```python
from build123d import *

# Parameters (mm, degrees)
F0_R     = 45.212
F1_DEPTH = 12.065
F2_R     = 2.5908
F3_DEPTH = 25.4
F4_R     = 14.5415
F5_DEPTH = 25.4
F6_R     = 6.731
F7_DEPTH = 9.525


with BuildPart() as f1:
    # F0 (on Top) → F1 (new body)
    with BuildSketch(Plane.XY):
        Circle(F0_R)
    extrude(amount=F1_DEPTH)

    # F2 (on face) → F3 (cut)
    with BuildSketch(Plane.XY.offset(12.065)):
        with Locations((-6.163129, 23.001109)):
            Circle(F2_R)
        with Locations((-23.001109, 6.163129)):
            Circle(F2_R)
        with Locations((-16.83798, -16.83798)):
            Circle(F2_R)
        with Locations((6.163129, -23.001109)):
            Circle(F2_R)
        with Locations((23.001109, -6.163129)):
            Circle(F2_R)
        with Locations((16.83798, 16.83798)):
            Circle(F2_R)
    extrude(amount=-F3_DEPTH, mode=Mode.SUBTRACT)

    # F4 (on face) → F5 (cut)
    with BuildSketch(Plane.XY.offset(12.065)):
        Circle(F4_R)
    extrude(amount=-F5_DEPTH, mode=Mode.SUBTRACT)

    # F6 (on face) → F7 (cut)
    with BuildSketch(Plane.XY.offset(12.065)):
        with Locations((-6.163129, 23.001109)):
            Circle(F6_R)
        with Locations((16.83798, 16.83798)):
            Circle(F6_R)
        with Locations((23.001109, -6.163129)):
            Circle(F6_R)
        with Locations((6.163129, -23.001109)):
            Circle(F6_R)
        with Locations((-16.83798, -16.83798)):
            Circle(F6_R)
        with Locations((-23.001109, 6.163129)):
            Circle(F6_R)
    extrude(amount=-F7_DEPTH, mode=Mode.SUBTRACT)


solid = f1.part
```
Could you check a few things on this model? Use its own coordinates, in mm. A direction names the side the tool comes from. Round coordinates to 2 decimals unless told otherwise and drop trailing zeros. Order: outer loops, then holes, each group sorted by start corner. A loop starts at its lowest first (then second) coordinate and runs counter-clockwise, first axis right, second up. Notation, with made-up numbers: (8.5, -2.75) -> (67.5, -2.75) arc R16 cw to (67.5, 3.25) -> close; hole circle Ø4 at (-21.5, -9). An arc over 180 degrees is marked (long way). One line per question, with ' | ' between items.
Q1. I'm going to push flat-ended pins straight in: pin 1 (8.5 mm diameter, centred on x = 16.84, y = 16.84, fed in from +Z); pin 2 (6 mm diameter, centred on y = -17.5, z = 4.5, fed in from +X); pin 3 (5 mm diameter, centred on x = -1, z = 8, fed in from +Y). Where does each tip first touch, or does it pass through?
Computed values:
pin 1: z = 2.54 | pin 2: x = 42.82 | pin 3: y = 45.21
Q2. If we section it at A-A on x = 22.5: Write out the boundary of the cut face in (y, z) (3 decimals).
Computed values:
outline: (-39.216, 0) -> (-8.705, 0) -> (-8.705, 2.54) -> (-12.875, 2.54) -> (-12.875, 12.065) -> (-39.216, 12.065) -> close; (-3.621, 0) -> (39.216, 0) -> (39.216, 12.065) -> (20.478, 12.065) -> (20.478, 2.54) -> (13.198, 2.54) -> (13.198, 12.065) -> (0.549, 12.065) -> (0.549, 2.54) -> (-3.621, 2.54) -> close
Q3. If we section it at B-B on z = 3.75: Write out the boundary of the cut face in (x, y).
Computed values:
outline: circle Ø90.42 at (0, 0); hole circle Ø13.46 at (-23, 6.16); hole circle Ø13.46 at (-16.84, -16.84); hole circle Ø29.08 at (0, 0); hole circle Ø13.46 at (-6.16, 23); hole circle Ø13.46 at (6.16, -23); hole circle Ø13.46 at (16.84, 16.84); hole circle Ø13.46 at (23, -6.16)
Q4. If I drill on line 1 (Y direction, x = -1.5, z = 6.25); line 2 (Y direction, x = 4, z = 11); line 3 (X direction, y = 8, z = 3.5), over which ranges is the centre line in solid material (lowest first)? Write a range as from..to.
Computed values:
line 1: -45.19..-14.46, 14.46..18.15, 27.86..45.19 | line 2: -45.03..-29.38, -16.63..-13.98, 13.98..45.03 | line 3: -44.5..-29.48, -16.53..-12.14, 12.14..44.5
Q5. If we section it at C-C on x = 5: Write out the boundary of the cut face in (y, z) (3 decimals), plus the area to 3 significant figures.
Computed values:
outline: (-44.935, 0) -> (-25.316, 0) -> (-25.316, 2.54) -> (-29.631, 2.54) -> (-29.631, 12.065) -> (-44.935, 12.065) -> close; (-20.686, 0) -> (-13.655, 0) -> (-13.655, 12.065) -> (-16.371, 12.065) -> (-16.371, 2.54) -> (-20.686, 2.54) -> close; (13.655, 0) -> (44.935, 0) -> (44.935, 12.065) -> (13.655, 12.065) -> close | area: 617 mm²
Q6. We'd pull the mould along X, two halves only. Please class faces 1 (the face through (43.124, 13.58, 5.948)), 2 (the face through (-17, -20, 2.54)), 3 (the face through (-11, 11, 12.065)): released by +X, released by -X, zero draft, split by the parting line, or undercut.
Computed values:
face 1: split by the parting line | face 2: undercut | face 3: zero draft
Q7. If we section it at D-D on y = -38.5: Write out the boundary of the cut face in (x, z) (3 decimals).
Computed values:
outline: (-23.704, 0) -> (23.704, 0) -> (23.704, 12.065) -> (-23.704, 12.065) -> close
Q8. Which directions (+Z, -Z, +X, -X, +Y, -Y) give clear straight access to the entire face, cutting with the end or side of a thin tool? Please do faces 4 (the face through (-14.445, -17.83, 1.288)), 5 (the face through (-7.039, 29.675, 7.369)).
Computed values:
face 4: +Z, -Z | face 5: +Z
